Input: part model. Units: mm. Frame: model coordinates. A direction names the side the tool comes from. Coordinates: 2 decimals unless noted, no trailing zeros. Order: outer loops, then holes, each group sorted by start corner. A loop starts at its lowest first (then second) coordinate and runs counter-clockwise, first axis right, second up. Notation, with made-up numbers: (75, 63.25) -> (111, 63.25) arc R8 ccw to (111, 70.25) -> close; hole circle Ø7 at (54.5, 56). An arc over 180 degrees is marked (long way). Answer as CSV lines item,"result".
from build123d import *

# Parameters (mm, degrees)
SKETCH_1_R               = 95
EXTRUDE_1_DEPTH          = 20
SKETCH_2_R               = 95
EXTRUDE_2_DEPTH          = 5
FILLET_1_R               = 5
SKETCH_5_R               = 1.5
CUT_EXTRUDE_2_DEPTH      = 137.656503775
CUT_EXTRUDE_9_DEPTH      = 136.830777142
CUT_EXTRUDE_9_DEPTH_BACK = 136.830777142


with BuildPart() as part:
    # 草圖1 → 填料-伸長1 (new body)
    with BuildSketch(Plane.XY):
        Circle(SKETCH_1_R)
        Polygon((64, 64), (-64, 64), (-64, 34.210333771), (-64, -34.210333771), (-64, -64), (64, -64), (64, -34.210333771), (64, 34.210333771), align=None, mode=Mode.SUBTRACT)
    extrude(amount=EXTRUDE_1_DEPTH)

    # 草圖2 → 填料-伸長2 (add)
    with BuildSketch(Plane.XY.offset(20)):
        Circle(SKETCH_2_R)
    extrude(amount=EXTRUDE_2_DEPTH)

    # 圓角1
    fillet_1_edges = [part.edges().sort_by_distance(p)[0] for p in [
        (-95, 0, 25),
    ]]
    fillet(fillet_1_edges, radius=FILLET_1_R)

    # 草圖5 → 除料-伸長2 (cut, through all)
    with BuildSketch(Plane(origin=(0, 0, 0), x_dir=(-1, 0, 0), z_dir=(0, 0, -1))):
        with Locations((-25, 75)):
            Circle(SKETCH_5_R)
        with Locations((25, 75)):
            Circle(SKETCH_5_R)
        with Locations((25, -75)):
            Circle(SKETCH_5_R)
        with Locations((-25, -75)):
            Circle(SKETCH_5_R)
    extrude(amount=-CUT_EXTRUDE_2_DEPTH, mode=Mode.SUBTRACT)

    # 草圖6 → 除料-伸長9 (cut, two sides: drawn at the far end of the back side and taken through both)
    with BuildSketch(Plane(origin=(0, 0, 20), x_dir=(-1, 0, 0), z_dir=(0, 0, -1)).offset(-CUT_EXTRUDE_9_DEPTH_BACK)):
        with BuildLine():
            Line((-64, 35), (-64, -35))
            Line((-64, -35), (-69, -35))
            ThreePointArc((-69, -35), (-72.535533906, -33.535533906), (-74, -30))
            Line((-74, -30), (-74, 30))
            ThreePointArc((-74, 30), (-72.535533906, 33.535533906), (-69, 35))
            Line((-69, 35), (-64, 35))
        make_face()
        with BuildLine():
            Line((64, -35), (69, -35))
            ThreePointArc((69, -35), (72.535533906, -33.535533906), (74, -30))
            Line((74, -30), (74, 30))
            ThreePointArc((74, 30), (72.535533906, 33.535533906), (69, 35))
            Line((69, 35), (64, 35))
            Line((64, 35), (64, -35))
        make_face()
    extrude(amount=CUT_EXTRUDE_9_DEPTH + CUT_EXTRUDE_9_DEPTH_BACK, mode=Mode.SUBTRACT)


solid = part.part
1. Contact query for flat-ended pins moving along their axis: pin 1 (2 mm diameter, centred on x = 45, y = -12.5, fed in from -Z); pin 2 (6 mm diameter, centred on y = 49, z = 10, fed in from -X); pin 3 (1 mm diameter, centred on x = 4.5, z = 18, fed in from +Y). Output: stop coordinate, or through.
Findings:
pin 1,"stops at z = 20"
pin 2,"stops at x = -83.12"
pin 3,"stops at y = 94.92"
2. Cut plane C-C (y = -20). State how many separate pieces and enclosed holes the cut face has, plus the area to 3 significant figures.
Findings:
separate pieces,"3"
enclosed holes,"0"
area,"1,570 mm2"
3. Mould query, pull axis X, two halves, no side actions, for faces 1 (the face through (7, 71, 0)), 2 (the face through (64, 50, 10)), 3 (the face through (72, -34, 13)), 4 (the face through (-20.59, -92.74, 9.86)). Classes: released by +X, released by -X, zero draft, split by the parting line, or undercut.
Findings:
face 1,"zero draft"
face 2,"undercut"
face 3,"undercut"
face 4,"split by the parting line"
4. Cut plane A-A (y = 0). Return the cut outline in (x, z).
Findings:
outline,"(-95, 0) -> (-74, 0) -> (-74, 25) -> (-90, 25) arc R5 ccw to (-95, 20) -> close; (-64, 20) -> (64, 20) -> (64, 25) -> (-64, 25) -> close; (74, 0) -> (95, 0) -> (95, 20) arc R5 ccw to (90, 25) -> (74, 25) -> close"
5. Cut plane B-B (z = 15.75). Return the cut outline in (x, y).
Findings:
outline,"circle Ø190 at (0, 0); hole (-74, -30) arc R5 ccw to (-69, -35) -> (-64, -35) -> (-64, -64) -> (64, -64) -> (64, -35) -> (69, -35) arc R5 ccw to (74, -30) -> (74, 30) arc R5 ccw to (69, 35) -> (64, 35) -> (64, 64) -> (-64, 64) -> (-64, 35) -> (-69, 35) arc R5 ccw to (-74, 30) -> close; hole circle Ø3 at (-25, -75); hole circle Ø3 at (-25, 75); hole circle Ø3 at (25, -75); hole circle Ø3 at (25, 75)"
6. Reachability of faces 5 (the face through (-1, 1, 20)), 6 (the face through (-1, 1, 25)), 7 (the face through (-67, 35, 13)) from +Z, -Z, +X, -X, +Y, -Y: full face, straight path, thin tool, end or side. Return the list, or none.
Findings:
face 5,"-Z"
face 6,"+Z, +X, -X, +Y, -Y"
face 7,"+Z, -Z"
7. Ray query, line 1 along X through (y, z) = (-75, 6); line 2 along Y through (x, z) = (-25, 15); line 3 along Z through (x, y) = (-35, -39). Return the intervals inside material, ascending.
Findings:
line 1,"x = -58.31 to -26.5, -23.5 to 23.5, 26.5 to 58.31"
line 2,"y = -91.65 to -76.5, -73.5 to -64, 64 to 73.5, 76.5 to 91.65"
line 3,"z = 20 to 25"
